```python
from build123d import *

# Parameters (mm, degrees)
F1_DEPTH = 4.5


# Not quite as in the source:
# - ends of sketch curves that miss each other by under 0.0002 mm in the source are joined


with BuildPart() as f1:
    # F0 (on Front) → F1 (new body, symmetric)
    with BuildSketch(Plane.XZ):
        with BuildLine():
            ThreePointArc((22.8784841202, 85.4427339913), (13.8060493669, 106.7545909747), (-1.20352e-05, 125.3528970532))
            ThreePointArc((-1.20352e-05, 125.3528970532), (-13.8060738367, 106.7545832167), (-22.8785085989, 85.4427260857))
            ThreePointArc((-22.8785085989, 85.4427260857), (-33.781429845, 94.2345199978), (-45.9220242093, 101.2184408782))
            ThreePointArc((-45.9220242093, 101.2184408782), (-49.5683429395, 87.6953665193), (-51.06114092, 73.7691058897))
            ThreePointArc((-51.06114092, 73.7691058897), (-72.5460800364, 82.4236845525), (-95.4594281867, 85.8123133595))
            ThreePointArc((-95.4594281867, 85.8123133595), (-92.0708001004, 62.8989646397), (-83.4162216453, 41.4140256538))
            ThreePointArc((-83.4162216453, 41.4140256538), (-97.3424818216, 39.9212276371), (-110.8655561911, 36.2749088727))
            ThreePointArc((-110.8655561911, 36.2749088727), (-103.8306945008, 24.0599857757), (-94.9659655862, 13.1005055314))
            ThreePointArc((-94.9659655862, 13.1005055314), (-109.3441086085, 8.1228594383), (-122.9337436667, 1.2796299938))
            ThreePointArc((-122.9337436667, 1.2796299938), (-124.3847743538, 0.5744976537), (-125.9303092338, 0.1118710562))
            ThreePointArc((-125.9303092338, 0.1118710562), (-134.5040813307, -0.8405705466), (-143.0970012567, -0.0800174007))
            ThreePointArc((-143.0970012567, -0.0800174007), (-90.2945054943, -33.7590284811), (-27.9154142382, -28.1707970164))
            ThreePointArc((-27.9154142382, -28.1707970164), (-21.9577774473, -32.956766848), (-15.1986970778, -36.5224048048))
            Line((-15.1986970778, -36.5224048048), (-15.1986972, -45.5224051023))
            Line((-15.1986972, -45.5224051023), (15.1986718, -45.5224051023))
            Line((15.1986718, -45.5224051023), (15.1986718, -36.5224051023))
            ThreePointArc((15.1986718, -36.5224051023), (21.9577523614, -32.9567672985), (27.9153889991, -28.1707973067))
            ThreePointArc((27.9153889991, -28.1707973067), (90.2944800943, -33.7590284811), (143.096975735, -0.0800170504))
            ThreePointArc((143.096975735, -0.0800170504), (134.5040559307, -0.8405705466), (125.9302837161, 0.1118705041))
            ThreePointArc((125.9302837161, 0.1118705041), (124.3847489538, 0.5744976537), (122.9337187314, 1.2796307814))
            ThreePointArc((122.9337187314, 1.2796307814), (109.3440836528, 8.1228592505), (94.9659404823, 13.1005047349))
            ThreePointArc((94.9659404823, 13.1005047349), (103.8306699794, 24.0599855987), (110.8655315962, 36.2749085192))
            ThreePointArc((110.8655315962, 36.2749085192), (97.3424564216, 39.9212276371), (83.416195792, 41.4140256177))
            ThreePointArc((83.416195792, 41.4140256177), (92.0707747004, 62.8989646397), (95.4594032906, 85.8123128836))
            ThreePointArc((95.4594032906, 85.8123128836), (72.5460546364, 82.4236845525), (51.0611157869, 73.7691059217))
            ThreePointArc((51.0611157869, 73.7691059217), (49.568318506, 87.695366698), (45.9219996628, 101.2184412045))
            ThreePointArc((45.9219996628, 101.2184412045), (33.7814018374, 94.2345137024), (22.8784841202, 85.4427339913))
        make_face()
        with BuildLine():
            ThreePointArc((-117.1095228717, -7.3640305351), (-89.448563488, 7.1418522166), (-58.5697361978, 11.837311045))
            ThreePointArc((-58.5697361978, 11.837311045), (-49.6119110254, 5.4631464022), (-39.9984925953, 0.1288430808))
            ThreePointArc((-39.9984925953, 0.1288430808), (-37.2748571799, -14.0339843315), (-29.705402075, -26.3102719896))
            ThreePointArc((-29.705402075, -26.3102719896), (-76.1944797379, -29.6944118928), (-117.1095228717, -7.3640305351))
        make_face(mode=Mode.SUBTRACT)
        with BuildLine():
            ThreePointArc((-91.0135912807, 14.1048128348), (-96.9513599422, 22.91124928), (-101.6267610462, 32.4480749604))
            ThreePointArc((-101.6267610462, 32.4480749604), (-91.6920273332, 35.8548732281), (-81.3873643524, 37.8844380956))
            ThreePointArc((-81.3873643524, 37.8844380956), (-73.7352473768, 26.9438563456), (-64.6715808547, 17.1407372042))
            ThreePointArc((-64.6715808547, 17.1407372042), (-77.9309186705, 16.3892197846), (-91.0135912807, 14.1048128348))
        make_face(mode=Mode.SUBTRACT)
        with BuildLine():
            ThreePointArc((-39.8747349061, 3.6409013815), (-70.812382671, 34.1134059196), (-84.8528261577, 75.2057109018))
            ThreePointArc((-84.8528261577, 75.2057109018), (-53.0294964681, 66.289674717), (-26.223286677, 46.9597204349))
            ThreePointArc((-26.223286677, 46.9597204349), (-25.1618451244, 39.8254262579), (-23.5802802502, 32.7881348844))
            ThreePointArc((-23.5802802502, 32.7881348844), (-34.9145400541, 19.9961948661), (-39.8747349061, 3.6409013815))
        make_face(mode=Mode.SUBTRACT)
        with BuildLine():
            ThreePointArc((58.569710798, 11.8373110298), (89.4485382345, 7.1418524965), (117.109497837, -7.3640300535))
            ThreePointArc((117.109497837, -7.3640300535), (76.1944543379, -29.6944118928), (29.7053768652, -26.3102719286))
            ThreePointArc((29.7053768652, -26.3102719286), (37.2748326568, -14.0339846476), (39.9984674303, 0.1288438922))
            ThreePointArc((39.9984674303, 0.1288438922), (49.6118856254, 5.4631464022), (58.569710798, 11.8373110298))
        make_face(mode=Mode.SUBTRACT)
        with BuildLine():
            ThreePointArc((-29.6372783208, -4.1734756121), (-2.3326090766, 30.3867739538), (29.9999878, 0.4775948977))
            ThreePointArc((29.9999878, 0.4775948977), (29.9091668501, -1.8550020562), (29.6372538967, -4.1734757653))
            ThreePointArc((29.6372538967, -4.1734757653), (-1.22775e-05, -29.5224051023), (-29.6372783208, -4.1734756121))
        make_face(mode=Mode.SUBTRACT)
        with BuildLine():
            ThreePointArc((26.2232617618, 46.9597209347), (53.0294713817, 66.2896748681), (84.8528008041, 75.2057108554))
            ThreePointArc((84.8528008041, 75.2057108554), (70.812357271, 34.1134059196), (39.8747095061, 3.6409013815))
            ThreePointArc((39.8747095061, 3.6409013815), (34.9145154377, 19.9961952532), (23.5802548967, 32.7881350301))
            ThreePointArc((23.5802548967, 32.7881350301), (25.161820701, 39.8254261326), (26.2232617618, 46.9597209347))
        make_face(mode=Mode.SUBTRACT)
        with BuildLine():
            ThreePointArc((81.3873389524, 37.8844380956), (91.6920019332, 35.8548732281), (101.6267360258, 32.4480754342))
            ThreePointArc((101.6267360258, 32.4480754342), (96.9513354477, 22.9112491166), (91.0135668807, 14.1048128348))
            ThreePointArc((91.0135668807, 14.1048128348), (77.930893754, 16.3892197289), (64.6715548016, 17.1407368356))
            ThreePointArc((64.6715548016, 17.1407368356), (73.7352219768, 26.9438563456), (81.3873389524, 37.8844380956))
        make_face(mode=Mode.SUBTRACT)
        with BuildLine():
            ThreePointArc((-47.3705884445, 71.6430268074), (-45.4199295453, 81.9895572502), (-42.0951898382, 91.9796457495))
            ThreePointArc((-42.0951898382, 91.9796457495), (-32.6613025725, 87.3636976735), (-23.9396864079, 81.5123196292))
            ThreePointArc((-23.9396864079, 81.5123196292), (-26.2649806939, 68.3652971805), (-26.7878526914, 55.0244649123))
            ThreePointArc((-26.7878526914, 55.0244649123), (-36.517789196, 64.0291013139), (-47.3705884445, 71.6430268074))
        make_face(mode=Mode.SUBTRACT)
        with BuildLine():
            ThreePointArc((-20.2364600157, 34.9810104129), (-18.2633780761, 74.8538230805), (-1.22419e-05, 110.352889417))
            ThreePointArc((-1.22419e-05, 110.352889417), (18.2633527585, 74.8538302889), (20.2364346157, 34.9810179281))
            ThreePointArc((20.2364346157, 34.9810179281), (-1.26313e-05, 40.4775948977), (-20.2364600157, 34.9810104129))
        make_face(mode=Mode.SUBTRACT)
        with BuildLine():
            ThreePointArc((23.9396582776, 81.5123130375), (32.6612744421, 87.3636910819), (42.0951621324, 91.9796391523))
            ThreePointArc((42.0951621324, 91.9796391523), (45.5019631468, 82.0449119699), (47.5315280138, 71.7402489249))
            ThreePointArc((47.5315280138, 71.7402489249), (36.5909469807, 64.0881318591), (26.7878276352, 55.0244650532))
            ThreePointArc((26.7878276352, 55.0244650532), (26.2649562826, 68.3652972858), (23.9396582776, 81.5123130375))
        make_face(mode=Mode.SUBTRACT)
    extrude(amount=F1_DEPTH, both=True)


solid = f1.part
```
Check sheet for the modelled part. Datum: model origin and axes. Units: mm. Coordinates: 2 decimals unless noted, no trailing zeros. Order: outer loops, then holes, each group sorted by start corner. A loop starts at its lowest first (then second) coordinate and runs counter-clockwise, first axis right, second up. Notation, with made-up numbers: (0, 55.5) -> (11, 55.5) arc R19 ccw to (11, 68.5) -> close; hole circle Ø4 at (33, 10). An arc over 180 degrees is marked (long way). Write item = value, one per line. Start each with the question number.
1) Cross-section at C-C (z = -19.5). Enter the section's corners in (x, y).
2) Material ranges on L1, parallel to X at y = 3.25, z = -24; L2, parallel to X at y = 3, z = -17; L3, parallel to Z at x = -106.5, y = -0.75, recorded low to high.
3) Go/stop test with flat-tipped pins: P1, Ø4.5, axis at y = -1, z = -39.5, coming from the +X side; P2, Ø4, axis at x = 85, y = -0.5, coming from the -Z side; P3, Ø1.5, axis at y = 0.5, z = 62.5, coming from the -X side; P4, Ø6, axis at x = 109.5, z = -4.5, coming from the +Y side. Record where each tip stops, or that it passes through.
4) Cross-section at B-B (z = 64.5). Enter the section's corners in (x, y), then the cut area to 3 significant figures.
5) Cross-section at A-A (x = -62). Enter the section's corners in (y, z).
6) Mould release check, pull along Z, two halves, no side actions. Record for faces 1 (the cylindrical face through (89.03, -0.06, 7.28)), 2 (the cylindrical face through (-22.047, -0.063, -32.898)), 3 (the cylindrical face through (-134.38, -0.06, -0.84)): +Z half, -Z half, draft (parallel to the pull), parting line (faces both ways), or undercut.
7) Cross-section at D-D (y = -2.5). State how many separate pieces and enclosed holes the cut face has, then the cut area to 3 significant figures.
Ans:
q1.outline = (-122.2, -4.5) -> (-101.68, -4.5) -> (-101.68, 4.5) -> (-122.2, 4.5) -> close; (-34.65, -4.5) -> (-22.38, -4.5) -> (-22.38, 4.5) -> (-34.65, 4.5) -> close; (22.38, -4.5) -> (34.65, -4.5) -> (34.65, 4.5) -> (22.38, 4.5) -> close; (101.68, -4.5) -> (122.2, -4.5) -> (122.2, 4.5) -> (101.68, 4.5) -> close
q2.L1 = -114.98 to -93.24, -31.64 to -17.34, 17.34 to 31.64, 93.24 to 114.98
q2.L2 = -125.68 to -105.54, -35.98 to -24.38, 24.38 to 35.98, 105.54 to 125.68
q2.L3 = -28.25 to -16.33, -0.39 to 9.28, 28.19 to 37.7
q3.P1 = 15.2
q3.P2 = -35.24
q3.P3 = -92.17
q3.P4 = 4.5
q4.outline = (-92.49, -4.5) -> (-83.18, -4.5) -> (-83.18, 4.5) -> (-92.49, 4.5) -> close; (-49.51, -4.5) -> (-37.11, -4.5) -> (-37.11, 4.5) -> (-49.51, 4.5) -> close; (-26.6, -4.5) -> (-20.43, -4.5) -> (-20.43, 4.5) -> (-26.6, 4.5) -> close; (20.43, -4.5) -> (26.6, -4.5) -> (26.6, 4.5) -> (20.43, 4.5) -> close; (37.11, -4.5) -> (49.51, -4.5) -> (49.51, 4.5) -> (37.11, 4.5) -> close; (83.18, -4.5) -> (92.49, -4.5) -> (92.49, 4.5) -> (83.18, 4.5) -> close
q4.area = 502 mm²
q5.outline = (-4.5, -36.38) -> (4.5, -36.38) -> (4.5, -31.5) -> (-4.5, -31.5) -> close; (-4.5, 11.83) -> (4.5, 11.83) -> (4.5, 22.26) -> (-4.5, 22.26) -> close; (-4.5, 70.06) -> (4.5, 70.06) -> (4.5, 78.91) -> (-4.5, 78.91) -> close
q6.face_1 = undercut
q6.face_2 = -Z half
q6.face_3 = +Z half
q7.separate_pieces = 1
q7.enclosed_holes = 10
q7.area = 9,900 mm²
